Read the model definition and answer for the solid it produces. Units are mm, in the model's axes. Face numbers are marked on the shaded views. A direction names the side the tool comes from. Give positions to 0.01 mm unless a question says otherwise; leave off trailing zeros. Loops run counter-clockwise (first coordinate to the right, second up) from the corner with the lowest first, then second, coordinate; pieces in that order, holes last. Notation, with made-up numbers: (54.25, 14) - (110.25, 14) arc R18 ccw to (110.25, 22) - close; hole circle Ø7 at (-4.5, -6). An arc over 180 degrees is marked (long way). Write each question's results on one line, items separated by ' | '. Start each with the question number.
Q1. The part is cut by section A-A, the plane x = 5. Write down the section's boundary in (y, z).
Q2. Find the intervals of material crossed by line 1 (Y direction, x = 1, z = -1.75); line 2 (X direction, y = 1.75, z = -1.5); line 3 (Z direction, x = 2, y = 10.25), in increasing order. Write a range as from..to.
Q3. For the marked faces 1 and 2, determine the directions among +Z, -Z, +X, -X, +Y, -Y from which every point of the face is accessible in a straight line to the end or side of a thin tool.
Q4. The part is cut by section B-B, the plane y = 7.25. Write down the section's boundary in (x, z), plus the area to 3 significant figures.
Q5. The part is cut by section D-D, the plane z = -6.75. Write down the section's boundary in (x, y), plus the area to 3 significant figures.
Q6. The part is cut by section C-C, the plane z = -4.5. Write down the section's boundary in (x, y), plus the area to 3 significant figures.
Q7. Given pin 1 (5 mm diameter, centred on x = 1, y = 2.5, fed in from -Z); pin 2 (1.5 mm diameter, centred on x = 9, y = 5, fed in from +Z); pin 3 (1.5 mm diameter, centred on y = 5, z = -5.5, fed in from +X), each flat-ended and moving along its own axis, determine where each tip first touches the part or whether it passes through.
```python
from build123d import *

# Parameters (mm, degrees)
BOSS_EXTRU_1_DEPTH = 12.5
ESQUISSE2_R        = 1.35
BOSS_EXTRU_2_DEPTH = 3


with BuildPart() as part:
    # Esquisse1 → Boss.-Extru.1 (new body)
    with BuildSketch(Plane(origin=(0, 0, 0), x_dir=(1, 0, 0), z_dir=(0, 1, 0))):
        with BuildLine():
            ThreePointArc((0, 4), (1.171572875, 1.171572875), (4, 0))
            Line((4, 0), (6, 0))
            ThreePointArc((6, 0), (8.828427125, 1.171572875), (10, 4))
            ThreePointArc((10, 4), (8.828427125, 6.828427125), (6, 8))
            Line((6, 8), (4, 8))
            ThreePointArc((4, 8), (1.171572875, 6.828427125), (0, 4))
        make_face()
    extrude(amount=BOSS_EXTRU_1_DEPTH)

    # Esquisse2 → Boss.-Extru.2 (add)
    with BuildSketch(Plane(origin=(0, 12.5, 0), x_dir=(1, 0, 0), z_dir=(0, 1, 0))):
        with Locations(Location((5, 4, 0), (0, 0, 270))):
            Circle(ESQUISSE2_R)
    extrude(amount=BOSS_EXTRU_2_DEPTH)


solid = part.part
```
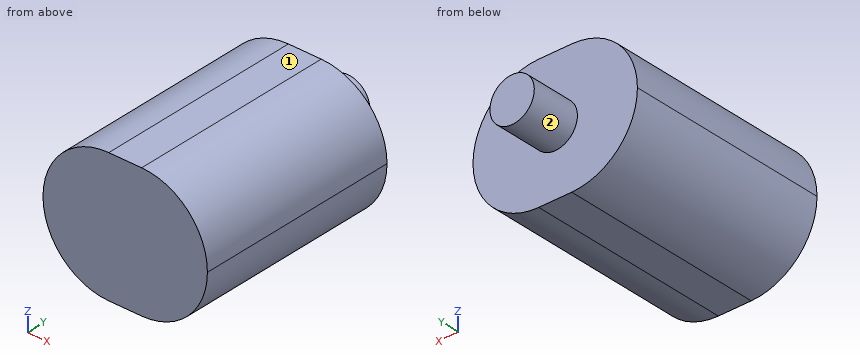
Check sheet entries:
1) outline: (0, -8) - (12.5, -8) - (12.5, -5.35) - (15.5, -5.35) - (15.5, -2.65) - (12.5, -2.65) - (12.5, 0) - (0, 0) - close
2) line 1: y = 0..12.5 | line 2: x = 0.88..9.12 | line 3: z = -7.46..-0.54
3) face 1: +Z, +X, -X, +Y, -Y | face 2: +Y
4) outline: (4, -8) - (6, -8) arc R4 ccw to (6, 0) - (4, 0) arc R4 ccw to start | area: 66.3 mm^2
5) outline: (1.1, 0) - (8.9, 0) - (8.9, 12.5) - (1.1, 12.5) - close | area: 97.6 mm^2
6) outline: (0.03, 0) - (9.97, 0) - (9.97, 12.5) - (6.25, 12.5) - (6.25, 15.5) - (3.75, 15.5) - (3.75, 12.5) - (0.03, 12.5) - close | area: 132 mm^2
7) pin 1: stops at z = -7.97 | pin 2: stops at z = -0.69 | pin 3: stops at x = 9.93
